```python
from build123d import *

# Parameters (mm, degrees)
EXTRUSION1_REACH                  = 105.556
EXTRUSION1_END_RADIUS             = 17.75
EXTRUSION1_DIRECTION_2_REACH      = 105.556
EXTRUSION1_DIRECTION_2_END_RADIUS = 17.75
CHANFREIN1_SIZE                   = 1
ESQUISSE3_R                       = 16.75
EXTRUSION2_DEPTH                  = 49
EXTRUSION3_START                  = -5
ESQUISSE6_R                       = 17.75
EXTRUSION3_DEPTH                  = 5
ESQUISSE8_R                       = 1.5
EXTRUSION4_DEPTH                  = 5


with BuildPart() as part:
    # Esquisse1 → Révolution1 (revolve)
    with BuildSketch(Plane.XY, mode=Mode.PRIVATE) as r_volution1_sk:
        Polygon((0, 0), (17.75, 0), (17.75, 49.6), (17.35, 49.6), (17.35, 54.6), (18.5, 54.596448784), (18.5, 79.196448784), (6, 79.196448784), (6, 85.196448784), (3, 85.196448784), (3, 100.196448784), (0, 100.196448784), align=None)
    revolve(r_volution1_sk.sketch.rotate(Axis((0, 100.196448784, 0), (0, -1, 0)), 90), axis=Axis((0, 100.196448784, 0), (0, -1, 0)))

    # Extrusion1: up to this cylinder (the profile starts inside it)
    extrusion1_end = Plane(origin=(0, 14.5, 0), z_dir=(0, 1, 0)) * Cylinder(EXTRUSION1_END_RADIUS, 247.612, mode=Mode.PRIVATE)
    # Esquisse2 → Extrusion1 (cut, up to the surface)
    with BuildSketch(Plane.XY, mode=Mode.PRIVATE) as extrusion1_sk1:
        with BuildLine():
            Line((-5.5, 17.5), (5.5, 17.5))
            ThreePointArc((5.5, 17.5), (8.5, 14.5), (5.5, 11.5))
            Line((5.5, 11.5), (-5.5, 11.5))
            ThreePointArc((-5.5, 11.5), (-8.5, 14.5), (-5.5, 17.5))
        make_face()
    extrusion1_tool1 = extrude(extrusion1_sk1.sketch, amount=EXTRUSION1_REACH, mode=Mode.PRIVATE) & extrusion1_end
    add(extrusion1_tool1.solids().sort_by_distance((0, 14.5, 0))[0], mode=Mode.SUBTRACT)

    # Extrusion1 direction 2: up to this cylinder (the profile starts inside it)
    extrusion1_direction_2_end = Plane(origin=(0, 14.5, 0), z_dir=(0, 1, 0)) * Cylinder(EXTRUSION1_DIRECTION_2_END_RADIUS, 247.612, mode=Mode.PRIVATE)
    # Esquisse2 → Extrusion1 direction 2 (cut, up to the surface)
    with BuildSketch(Plane.XY, mode=Mode.PRIVATE) as extrusion1_direction_2_sk1:
        with BuildLine():
            Line((-5.5, 17.5), (5.5, 17.5))
            ThreePointArc((5.5, 17.5), (8.5, 14.5), (5.5, 11.5))
            Line((5.5, 11.5), (-5.5, 11.5))
            ThreePointArc((-5.5, 11.5), (-8.5, 14.5), (-5.5, 17.5))
        make_face()
    extrusion1_direction_2_tool1 = extrude(extrusion1_direction_2_sk1.sketch, amount=-EXTRUSION1_DIRECTION_2_REACH, mode=Mode.PRIVATE) & extrusion1_direction_2_end
    add(extrusion1_direction_2_tool1.solids().sort_by_distance((0, 14.5, 0))[0], mode=Mode.SUBTRACT)

    # Chanfrein1
    chanfrein1_edges = [part.edges().sort_by_distance(p)[0] for p in [
        (0, 85.196448784, -6),
    ]]
    chamfer(chanfrein1_edges, length=CHANFREIN1_SIZE)

    # Esquisse3 → Extrusion2 (cut)
    with BuildSketch(Plane.XZ):
        with Locations(Location((0, 0, 0), (0, 0, 270))):
            Circle(ESQUISSE3_R)
    extrude(amount=-EXTRUSION2_DEPTH, mode=Mode.SUBTRACT)

    # Esquisse6 → Extrusion3 (add)
    with BuildSketch(Plane.XZ.offset(EXTRUSION3_START)):
        with Locations(Location((0, 0, 0), (0, 0, 90))):
            Circle(ESQUISSE6_R)
    extrude(amount=EXTRUSION3_DEPTH)

    # Esquisse8 → Extrusion4 (cut)
    with BuildSketch(Plane(origin=(0, 79.196448784, 0), x_dir=(-1, 0, 0), z_dir=(0, 1, 0))):
        with Locations(Location((15, 0, 0), (0, 0, 90))):
            Circle(ESQUISSE8_R)
        with Locations(Location((-7.5, -12.990381057, 0), (0, 0, 90))):
            Circle(ESQUISSE8_R)
        with Locations(Location((-7.5, 12.990381057, 0), (0, 0, 90))):
            Circle(ESQUISSE8_R)
    extrude(amount=-EXTRUSION4_DEPTH, mode=Mode.SUBTRACT)


solid = part.part
```
Part model, mm, in its own coordinate system. A direction names the side the tool comes from. Round coordinates to 2 decimals unless told otherwise and drop trailing zeros. Write each loop counter-clockwise with the first axis right and the second up, starting at its lowest first coordinate (ties: lowest second). Pieces come first, ordered by that corner, then holes.
Item 1: Cut at C-C, the plane y = 14.5. Give the cut face in (x, z), plus the area to 3 significant figures.
Results:
outline: (-8.5, -15.58) - (-8.5, -14.43) arc R16.75 cw to (-8.5, 14.43) - (-8.5, 15.58) arc R17.75 ccw to start; (8.5, -15.58) arc R17.75 ccw to (8.5, 15.58) - (8.5, 14.43) arc R16.75 cw to (8.5, -14.43) - close
area: 72.8 mm2
Item 2: Which spindle directions (+Z, -Z, +X, -X, +Y, -Y) get a long thin tool onto all of the face, cutting with end or side? Do faces 5 (the flat face through (0, 0, 0)), 6 (the cylindrical face through (16.41, 67.07, 8.54)), 7 (the flat face through (0, 17.5, 17)), 8 (the cylindrical face through (6.587, 76.731, -14.181)), 9 (the cylindrical face through (0.736, 26.692, 16.734)). Say none if no direction does.
Results:
face 5: +Z, -Z, +X, -X, -Y
face 6: +Y, -Y
face 7: +Z, -Z
face 8: +Y
face 9: none
Item 3: Two-plate mould, pull along Y, no slides. Class faces 1 (the cylindrical face through (8.5, 14.6, 15.4)), 2 (the flat face through (0, 11.5, 17)), 3 (the cylindrical face through (6.17, 76.73, 13.68)), 4 (the flat face through (-15, 74.196, 0)): +Y half, -Y half, draft (parallel to the pull), parting line (faces both ways), or undercut.
Results:
face 1: undercut
face 2: undercut
face 3: draft
face 4: +Y half
Item 4: Probe L1, parallel to Y at x = 2.5, z = 5.5; L2, parallel to X at y = 77.5, z = 0; L3, parallel to X at y = 57.5, z = -11.5. List the from-to ranges inside material, lowest first.
Results:
L1: y = 0 to 5, 49 to 79.2
L2: x = -18.5 to -16.5, -13.5 to 18.5
L3: x = -14.49 to 14.49
Item 5: Cut at D-D, the plane y = 92. Give the cut face in (x, z).
Results:
outline: circle Ø6 at (0, 0)
Item 6: Drop flat-ended pins along their axis: pin 1 Ø3.5 at (x, z) = (7.5, 12.99) entering from +Y; pin 2 Ø11 at (x, z) = (-3.5, 3.5) entering from +Y; pin 3 Ø10 at (x, y) = (-12, 37) entering from -Z; pin 4 Ø4 at (x, z) = (-1.5, 6) entering from +Y. Give the stop position or say it passes through.
Results:
pin 1: stops at y = 79.2
pin 2: stops at y = 100.2
pin 3: stops at z = -16.31
pin 4: stops at y = 85.2
